Part model, mm, in its own coordinate system. A direction names the side the tool comes from. Round coordinates to 2 decimals unless told otherwise and drop trailing zeros. Loops run counter-clockwise (first coordinate to the right, second up) from the corner with the lowest first, then second, coordinate; pieces in that order, holes last. Notation, with made-up numbers: M 42,88 L 81,88 A11 cw 81,105 Z; hole C 27.5,87 d8. An arc over 180 degrees is marked long. Put each result on its own line as item: value. Start each with the question number.
1) Pull direction Y, two halves, no side cores. Call faces 1 (the flat face through (29, 14.01, 6)), 2 (the cylindrical face through (6.3, 6.1, 0.5)), 3 (the flat face through (14.5, 11, 2)): +Y half, -Y half, draft (parallel to the pull), parting line (faces both ways), or undercut.
2) Slice it at C-C on x = 23.5. Give the cut face in (y, z), then the cut area to 4 significant figures.
3) Which spindle directions (+Z, -Z, +X, -X, +Y, -Y) get a long thin tool onto all of the face, cutting with end or side? Do faces 4 (the flat face through (23, 13, 2)), 5 (the flat face through (11.1, 12, 1.5)), 6 (the flat face through (23, 12, 1.5)). Say none if no direction does.
4) Drop flat-ended pins along their axis: pin 1 Ø0.8 at (x, z) = (6.5, 1.5) entering from -Y; pin 2 Ø6 at (x, z) = (21.5, 5.5) entering from -Y. Give the stop position or say it passes through.
5) Probe line 1 along Y through (x, z) = (2, 0.85) (3 decimals); line 2 along Y through (x, z) = (27.5, 6.75); line 3 along Z through (x, y) = (9, 12). List the from-to ranges inside material, lowest first.
6) Slice it at A-A on z = 10. Give the cut face in (x, y).
```python
from build123d import *

# Parameters (mm, degrees)
ESQUISSE1_W        = 32
ESQUISSE1_H        = 14
ESQUISSE1_R        = 0.375
ESQUISSE1_R_2      = 1.5
BOSS_EXTRU_1_DEPTH = 1
ESQUISSE2_W        = 6
ESQUISSE2_H        = 14.02
BOSS_EXTRU_2_DEPTH = 2
ESQUISSE3_W        = 6
ESQUISSE3_H        = 4
BOSS_EXTRU_3_DEPTH = 8
ESQUISSE4_W        = 4
ESQUISSE4_H        = 5
BOSS_EXTRU_4_DEPTH = 1.5
ESQUISSE5_W        = 1.25
ESQUISSE5_H        = 2
ESQUISSE5_W_2      = 2
ESQUISSE5_H_2      = 1.25
BOSS_EXTRU_5_DEPTH = 1


with BuildPart() as part:
    # Esquisse1 → Boss.-Extru.1 (new body)
    with BuildSketch(Plane.XY):
        with Locations((16, 7)):
            Rectangle(ESQUISSE1_W, ESQUISSE1_H)
        with Locations((2, 8.25)):
            Circle(ESQUISSE1_R, mode=Mode.SUBTRACT)
        with Locations((2, 10.75)):
            Circle(ESQUISSE1_R, mode=Mode.SUBTRACT)
        with Locations((2, 5.75)):
            Circle(ESQUISSE1_R, mode=Mode.SUBTRACT)
        with Locations((2, 3.25)):
            Circle(ESQUISSE1_R, mode=Mode.SUBTRACT)
        with Locations((7.5, 7)):
            Circle(ESQUISSE1_R_2, mode=Mode.SUBTRACT)
    extrude(amount=BOSS_EXTRU_1_DEPTH)

    # Esquisse2 → Boss.-Extru.2 (add)
    with BuildSketch(Plane.XY.offset(1)):
        with Locations((29.01, 7)):
            Rectangle(ESQUISSE2_W, ESQUISSE2_H)
    extrude(amount=BOSS_EXTRU_2_DEPTH)

    # Esquisse3 → Boss.-Extru.3 (add)
    with BuildSketch(Plane.XY.offset(3)):
        with Locations((29.01, 12.01)):
            Rectangle(ESQUISSE3_W, ESQUISSE3_H)
        with Locations((29.01, 1.99)):
            Rectangle(ESQUISSE3_W, ESQUISSE3_H)
    extrude(amount=BOSS_EXTRU_3_DEPTH)

    # Esquisse4 → Boss.-Extru.4 (add)
    with BuildSketch(Plane.XY.offset(1)):
        with Locations((16.5, 11)):
            Rectangle(ESQUISSE4_W, ESQUISSE4_H)
    extrude(amount=BOSS_EXTRU_4_DEPTH)

    # Esquisse5 → Boss.-Extru.5 (add)
    with BuildSketch(Plane.XY.offset(1)):
        with Locations((11.125, 11)):
            Rectangle(ESQUISSE5_W, ESQUISSE5_H)
        with Locations((10.625, 3)):
            Rectangle(ESQUISSE5_W, ESQUISSE5_H)
        with Locations((14.125, 4)):
            Rectangle(ESQUISSE5_W, ESQUISSE5_H)
        with Locations((17.875, 4)):
            Rectangle(ESQUISSE5_W, ESQUISSE5_H)
        with Locations((23.01, 12.625)):
            Rectangle(ESQUISSE5_W_2, ESQUISSE5_H_2)
        with Locations((23.01, 9.875)):
            Rectangle(ESQUISSE5_W_2, ESQUISSE5_H_2)
        with Locations((23.01, 7.125)):
            Rectangle(ESQUISSE5_W_2, ESQUISSE5_H_2)
        with Locations((23.01, 4.375)):
            Rectangle(ESQUISSE5_W_2, ESQUISSE5_H_2)
        with Locations((23.01, 1.625)):
            Rectangle(ESQUISSE5_W_2, ESQUISSE5_H_2)
        with Locations((6.5, 12.375)):
            Rectangle(ESQUISSE5_W_2, ESQUISSE5_H_2)
        with Locations((6.5, 1.625)):
            Rectangle(ESQUISSE5_W_2, ESQUISSE5_H_2)
    extrude(amount=BOSS_EXTRU_5_DEPTH)


solid = part.part
```
Recorded:
1. face 1: +Y half
1. face 2: undercut
1. face 3: draft
2. outline: M 0,0 L 14,0 L 14,1 L 13.25,1 L 13.25,2 L 12,2 L 12,1 L 10.5,1 L 10.5,2 L 9.25,2 L 9.25,1 L 7.75,1 L 7.75,2 L 6.5,2 L 6.5,1 L 5,1 L 5,2 L 3.75,2 L 3.75,1 L 2.25,1 L 2.25,2 L 1,2 L 1,1 L 0,1 Z
2. area: 20.25 mm2
3. face 4: +Z, +Y, -Y
3. face 5: +Z, +Y
3. face 6: +Z
4. pin 1: stops at y = 1
4. pin 2: passes through
5. line 1: y = 0 to 2.875, 3.625 to 5.375, 6.125 to 7.875, 8.625 to 10.375, 11.125 to 14
5. line 2: y = -0.01 to 3.99, 10.01 to 14.01
5. line 3: z = 0 to 1
6. outline: M 26.01,-0.01 L 32.01,-0.01 L 32.01,3.99 L 26.01,3.99 Z; M 26.01,10.01 L 32.01,10.01 L 32.01,14.01 L 26.01,14.01 Z
